Can you work these out from the drawing? Everything is in mm from the part's minimum corner. A direction names the side the tool comes from. Give positions to 0.01 mm unless a question says otherwise; leave off trailing zeros. Order: outer loops, then holes, each group sorted by start corner. A loop starts at its lowest first (then second) coordinate and runs counter-clockwise, first axis right, second up. Notation, with made-up numbers: (26.25, 25.5) - (56.25, 25.5) arc R16 cw to (56.25, 31.5) - close; hole circle Ø9 at (-8.75, 81.25). An arc over 180 degrees is marked (long way). One line per question, with ' | ' between items.
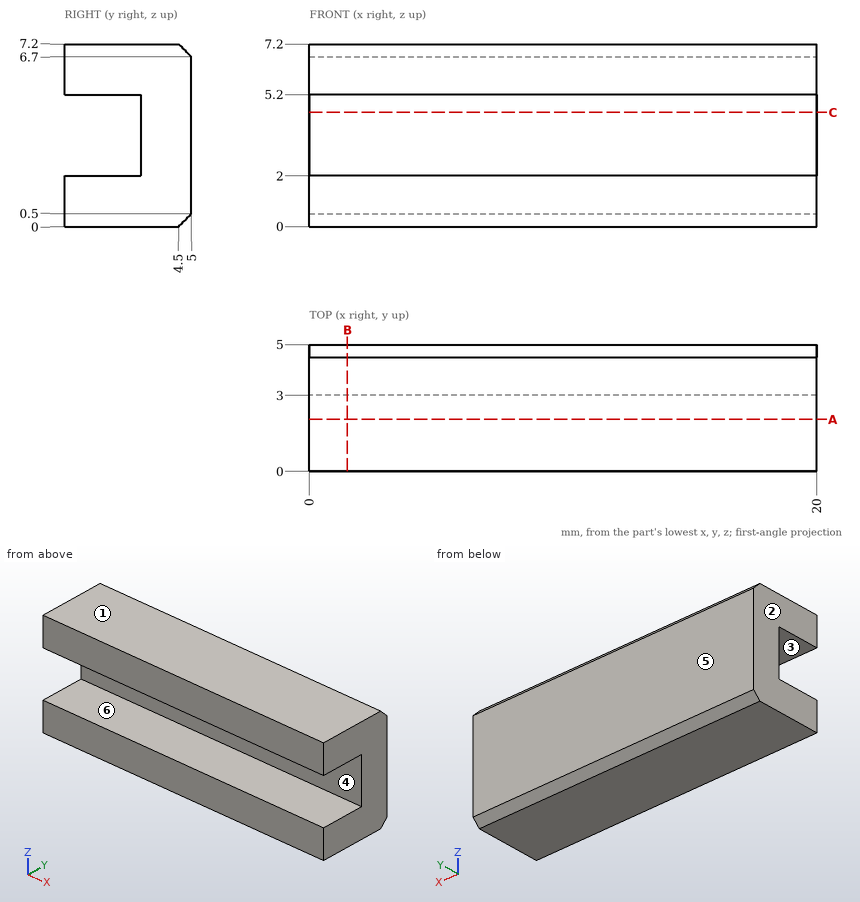
(1) Imagine slicing it at B-B (x = 1.5). List the corners of the cut face in (y, z) for me, and give its area (4 significant figures).
Answer below:
outline: (0, 0) - (4.5, 0) - (5, 0.5) - (5, 6.7) - (4.5, 7.2) - (0, 7.2) - (0, 5.2) - (3, 5.2) - (3, 2) - (0, 2) - close | area: 26.15 mm^2
(2) Imagine slicing it at A-A (y = 2.05). List the corners of the cut face in (x, z) for me, and give its area (3 significant figures).
Answer below:
outline: (0, 0) - (20, 0) - (20, 2) - (0, 2) - close; (0, 5.2) - (20, 5.2) - (20, 7.2) - (0, 7.2) - close | area: 80.0 mm^2
(3) Imagine slicing it at C-C (z = 4.5). List the corners of the cut face in (x, y) for me, and give its area (3 significant figures).
Answer below:
outline: (0, 3) - (20, 3) - (20, 5) - (0, 5) - close | area: 40.0 mm^2
(4) If we mould it in two halves opening along Z, with no side actions, what happens to the marked faces 1, 2, 3 and 4? For each: released by +Z, released by -Z, zero draft, split by the parting line, or undercut.
Answer below:
face 1: released by +Z | face 2: zero draft | face 3: undercut | face 4: undercut
(5) On a 3-axis mill with a long thin cutter (end or side, diameter ignored), from which of +Z, -Z, +X, -X, +Y, -Y can I reach the whole of each face in a straight line? I mean the marked faces 5 and 6. Say none if no direction works.
Answer below:
face 5: +Z, -Z, +X, -X, +Y | face 6: +X, -X, -Y
(6) If I drill on line 1 (Z direction, x = 11.5, y = 2.5); line 2 (Y direction, x = 12.5, z = 4.5), over which ranges is the centre line in solid material (lowest first)?
Answer below:
line 1: 0 to 2, 5.2 to 7.2 | line 2: 3 to 5
(7) Will these pins go through, and if not, where does the flat tip stop? pin 1 (4 mm diameter, centred on x = 10, z = 1.5, fed in from -Y); pin 2 (2.5 mm diameter, centred on x = 11, z = 3.5, fed in from -Y).
Answer below:
pin 1: y = 0 | pin 2: y = 3
